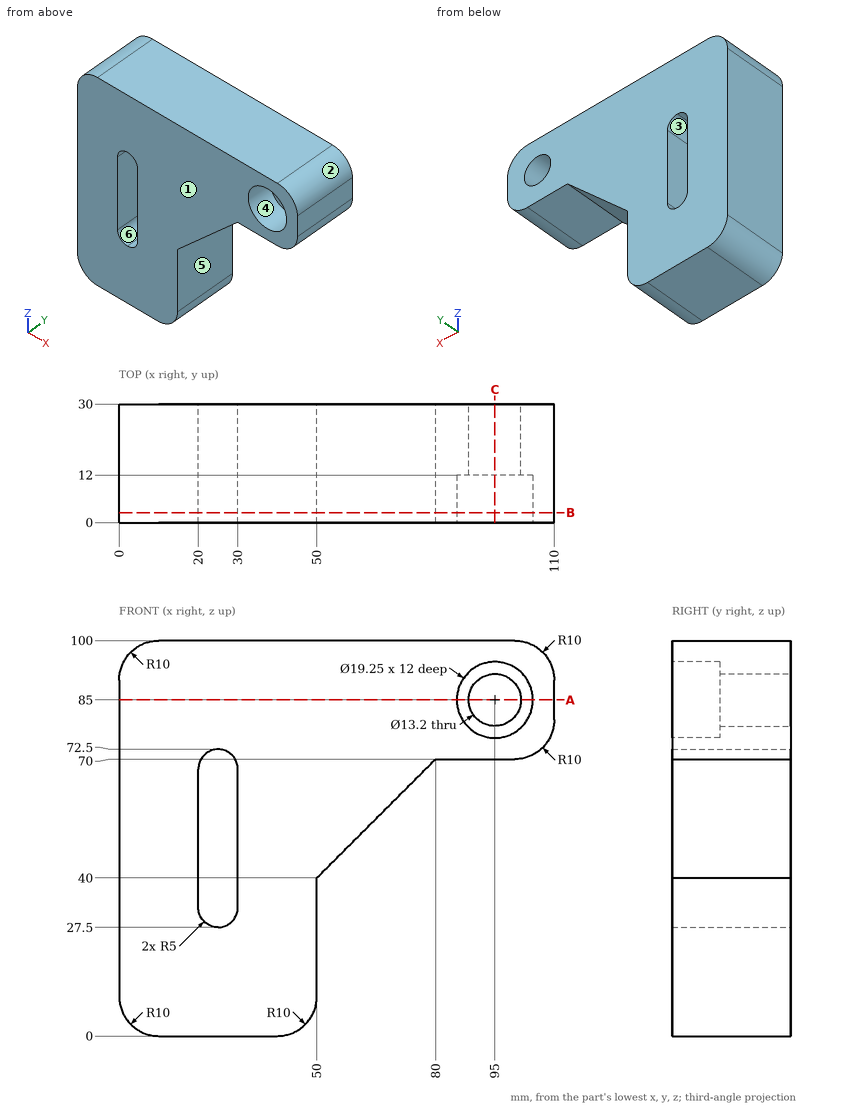
Verification items for this drawing (mm, ordinates from the low corner). A direction names the side the tool comes from. Coordinates: 2 decimals unless noted, no trailing zeros. Loops run counter-clockwise (first coordinate to the right, second up) from the corner with the lowest first, then second, coordinate; pieces in that order, holes last. Notation, with made-up numbers: (87.5, -38) -> (134.5, -38) arc R27 cw to (134.5, -18) -> close; hole circle Ø6 at (38.25, 57). An arc over 180 degrees is marked (long way). Answer in a Markdown table with one row per item. Add a question column.
1. Section check B-B, the plane y = 2.5. Give the number of separate pieces and of enclosed holes in the cut face, then the cut area to 3 significant figures.
2. Material ranges on probe 1 along Z at (x, y) = (95, 6.25) (3 decimals); probe 2 along Z at (x, y) = (95, 17.25); probe 3 along X at (y, z) = (19.5, 36), recorded low to high. Write a range as [from, to].
3. Access from +Z, -Z, +X, -X, +Y, -Y to the whole of each face (thin tool, end or side, straight path). Record for the marked faces 4, 5 and 6.
4. Depth check by flat-ended pin: P1, Ø5, axis at y = 12.5, z = 41.5, coming from the +X side; P2, Ø15, axis at y = 17.5, z = 23.5, coming from the +X side; P3, Ø9, axis at y = 21.5, z = 41.5, coming from the +X side. Enter the tip coordinate at first touch or a pass-through.
5. Draft check along X on the marked faces 1, 2 and 3. Enter one of: +X half, -X half, draft (parallel to the pull), parting line (faces both ways), or undercut.
6. Section check C-C, the plane x = 95. Enter the section's corners in (y, z) (3 decimals), then the cut area to 3 significant figures.
7. Section check A-A, the plane z = 85. Enter the section's corners in (x, y) (3 decimals), then the cut area to 3 significant figures.
Derived:
| question | item | result |
|---|---|---|
| 1 | separate pieces | 1 |
| 1 | enclosed holes | 2 |
| 1 | area | 6,420 mm² |
| 2 | probe 1 | z = [70, 75.375], [94.625, 100] |
| 2 | probe 2 | z = [70, 78.4], [91.6, 100] |
| 2 | probe 3 | x = [0, 20], [30, 50] |
| 3 | face 4 | -Y |
| 3 | face 5 | -Z, +X, +Y, -Y |
| 3 | face 6 | +Y, -Y |
| 4 | P1 | stops at x = 54 |
| 4 | P2 | stops at x = 50 |
| 4 | P3 | stops at x = 56 |
| 5 | face 1 | draft |
| 5 | face 2 | +X half |
| 5 | face 3 | undercut |
| 6 | outline | (0, 70) -> (30, 70) -> (30, 78.4) -> (12, 78.4) -> (12, 75.375) -> (0, 75.375) -> close; (0, 94.625) -> (12, 94.625) -> (12, 91.6) -> (30, 91.6) -> (30, 100) -> (0, 100) -> close |
| 6 | area | 431 mm² |
| 7 | outline | (0, 0) -> (85.375, 0) -> (85.375, 12) -> (88.4, 12) -> (88.4, 30) -> (0, 30) -> close; (101.6, 12) -> (104.625, 12) -> (104.625, 0) -> (110, 0) -> (110, 30) -> (101.6, 30) -> close |
| 7 | area | 2,830 mm² |
